Source: CAD feature listing. Evaluate the final solid. Frame: model axes, mm. A direction names the side the tool comes from. Give positions to 0.01 mm unless a question says otherwise; leave off trailing zeros. Order: outer loops, then holes, each group sorted by start corner. A loop starts at its lowest first (then second) coordinate and runs counter-clockwise, first axis right, second up. Notation, with made-up numbers: (-32, 43.5) -> (-15, 43.5) arc R13 ccw to (-15, 57.5) -> close; hole circle Ø5 at (12.25, 25.5). An arc over 180 degrees is marked (long way). Answer in a Markdown table with one row per item.
```python
from build123d import *

# Parameters (mm, degrees)
F0_W     = 127
F0_H     = 127
F1_DEPTH = 12.7
F2_R     = 4.826
F3_DEPTH = 25.4
F4_R     = 3.429
F4_R_2   = 3.4577066483
F5_DEPTH = 25.4


# Not quite as in the source:
# - a feature names something its author has since deleted; it is built from what else it names


with BuildPart() as f1:
    # F0 (on Top) → F1 (new body)
    with BuildSketch(Plane.XY):
        Rectangle(F0_W, F0_H)
    extrude(amount=F1_DEPTH)

    # F2 (on face) → F3 (cut)
    with BuildSketch(Plane.XY.offset(12.7)):
        with BuildLine():
            ThreePointArc((-10.8373346815, 7.9672162229), (-15.8950533343, 8.195276323), (-15.6669932342, 3.1375576702))
            ThreePointArc((-15.6669932342, 3.1375576702), (-12.0167906073, 2.664949958), (-10.0413841816, 5.7706071703))
            ThreePointArc((-10.0413841816, 5.7706071703), (-10.2465070332, 6.9387925717), (-10.8373346815, 7.9672162229))
        make_face()
        with BuildLine():
            ThreePointArc((3.429, 11.3502229887), (-0.1544617901, 14.7757423005), (-3.4150843134, 11.0416129887))
            ThreePointArc((-3.4150843134, 11.0416129887), (0, 7.9212229887), (3.4150843134, 11.0416129887))
            ThreePointArc((3.4150843134, 11.0416129887), (3.4255193118, 11.1957611986), (3.429, 11.3502229887))
        make_face()
        with BuildLine():
            ThreePointArc((16.8993841816, 5.7706071703), (14.638569583, 8.9944843187), (10.8373346815, 7.9672162229))
            ThreePointArc((10.8373346815, 7.9672162229), (11.0457150289, 3.3459380176), (15.6669932342, 3.1375576702))
            ThreePointArc((15.6669932342, 3.1375576702), (16.576041394, 4.317013596), (16.8993841816, 5.7706071703))
        make_face()
        with BuildLine():
            ThreePointArc((22.479, -7.6997770113), (21.3629869552, -5.1683480976), (18.74139, -4.2846926978))
            ThreePointArc((18.74139, -4.2846926978), (15.621, -7.6997770113), (18.74139, -11.1148613247))
            ThreePointArc((18.74139, -11.1148613247), (21.3629869552, -10.231205925), (22.479, -7.6997770113))
        make_face()
        with BuildLine():
            ThreePointArc((15.6669932342, -18.5371116928), (11.0457150289, -18.7454920402), (10.8373346815, -23.3667702455))
            ThreePointArc((10.8373346815, -23.3667702455), (14.638569583, -24.3940383413), (16.8993841816, -21.1701611929))
            ThreePointArc((16.8993841816, -21.1701611929), (16.576041394, -19.7165676186), (15.6669932342, -18.5371116928))
        make_face()
        with BuildLine():
            ThreePointArc((3.4150843134, -26.4411670113), (0, -23.3207770113), (-3.4150843134, -26.4411670113))
            ThreePointArc((-3.4150843134, -26.4411670113), (-0.1544617901, -30.1752963231), (3.429, -26.7497770113))
            ThreePointArc((3.429, -26.7497770113), (3.4255193118, -26.5953152212), (3.4150843134, -26.4411670113))
        make_face()
        with BuildLine():
            ThreePointArc((-10.0413841816, -21.1701611929), (-12.0167906073, -18.0645039805), (-15.6669932342, -18.5371116928))
            ThreePointArc((-15.6669932342, -18.5371116928), (-15.8950533343, -23.5948303456), (-10.8373346815, -23.3667702455))
            ThreePointArc((-10.8373346815, -23.3667702455), (-10.2465070332, -22.3383465943), (-10.0413841816, -21.1701611929))
        make_face()
        with BuildLine():
            ThreePointArc((-15.621, -7.6997770113), (-16.5185710863, -5.3867900561), (-18.74139, -4.2846926978))
            ThreePointArc((-18.74139, -4.2846926978), (-22.479, -7.6997770113), (-18.74139, -11.1148613247))
            ThreePointArc((-18.74139, -11.1148613247), (-16.5185710863, -10.0127639665), (-15.621, -7.6997770113))
        make_face()
        with Locations((0, -7.6997770113)):
            Circle(F2_R)
    extrude(amount=-F3_DEPTH, mode=Mode.SUBTRACT)

    # F4 (on face) → F5 (cut)
    with BuildSketch(Plane.XY.offset(12.7)):
        with Locations((0, 50.8)):
            Circle(F4_R)
        with Locations((27.94, -55.88)):
            Circle(F4_R)
        with Locations((50.8, -55.88)):
            Circle(F4_R)
        with Locations((-50.8, -55.88)):
            Circle(F4_R)
        with Locations((-27.94, -55.88)):
            Circle(F4_R)
        with Locations((-53.594, 50.8)):
            Circle(F4_R_2)
        with Locations((53.594, 50.8)):
            Circle(F4_R_2)
        with BuildLine():
            Line((-22.479, 54.229), (-35.814, 54.229))
            ThreePointArc((-35.814, 54.229), (-39.243, 50.8), (-35.814, 47.371))
            Line((-35.814, 47.371), (-22.479, 47.371))
            ThreePointArc((-22.479, 47.371), (-19.05, 50.8), (-22.479, 54.229))
        make_face()
        with BuildLine():
            ThreePointArc((35.814, 47.371), (39.243, 50.8), (35.814, 54.229))
            Line((35.814, 54.229), (22.479, 54.229))
            ThreePointArc((22.479, 54.229), (19.05, 50.8), (22.479, 47.371))
            Line((22.479, 47.371), (35.814, 47.371))
        make_face()
    extrude(amount=-F5_DEPTH, mode=Mode.SUBTRACT)


solid = f1.part
```
(1) Section query D-D (x = 20.5). Return the cut outline in (y, z), plus the area to 3 significant figures.
A:
| item | result |
|---|---|
| outline | (-63.5, 0) -> (-10.81, 0) -> (-10.81, 12.7) -> (-63.5, 12.7) -> close; (-4.59, 0) -> (48, 0) -> (48, 12.7) -> (-4.59, 12.7) -> close; (53.6, 0) -> (63.5, 0) -> (63.5, 12.7) -> (53.6, 12.7) -> close |
| area | 1,460 mm^2 |
(2) Access query for faces 5 (the flat face through (63.5, -1, 6)), 6 (the cylindrical face through (39.242, 50.725, 6.439)). Directions: +Z, -Z, +X, -X, +Y, -Y. A direction counts if a zero-diameter tool reaches every point of the face in a straight line with its end or side. Return the directions, or none.
A:
| item | result |
|---|---|
| face 5 | +Z, -Z, +X, +Y, -Y |
| face 6 | +Z, -Z |
(3) First-contact query: pin 1 Ø5.5 at (x, y) = (53.594, 50.8) entering from +Z. Flat tip, straight axial feed; report the tip coordinate or a pass-through.
A:
| item | result |
|---|---|
| pin 1 | passes through |
(4) Pull-direction query (Y, two-part tool) for faces 1 (the flat face through (-1, -63.5, 6)), 2 (the cylindrical face through (-28.39, -52.48, 6.44)), 3 (the flat face through (-63.5, -1, 6)), 4 (the flat face through (-1, 63.5, 6)); classes: +Y half, -Y half, draft (parallel to the pull), parting line (faces both ways), or undercut.
A:
| item | result |
|---|---|
| face 1 | -Y half |
| face 2 | undercut |
| face 3 | draft |
| face 4 | +Y half |
(5) Section query C-C (y = 50.8). Return the cut outline in (x, z), plus the area to 3 significant figures.
A:
| item | result |
|---|---|
| outline | (-63.5, 0) -> (-57.05, 0) -> (-57.05, 12.7) -> (-63.5, 12.7) -> close; (-50.14, 0) -> (-39.24, 0) -> (-39.24, 12.7) -> (-50.14, 12.7) -> close; (-19.05, 0) -> (-3.43, 0) -> (-3.43, 12.7) -> (-19.05, 12.7) -> close; (3.43, 0) -> (19.05, 0) -> (19.05, 12.7) -> (3.43, 12.7) -> close; (39.24, 0) -> (50.14, 0) -> (50.14, 12.7) -> (39.24, 12.7) -> close; (57.05, 0) -> (63.5, 0) -> (63.5, 12.7) -> (57.05, 12.7) -> close |
| area | 837 mm^2 |
(6) Section query A-A (x = 0). Return the cut outline in (y, z), plus the area to 3 significant figures.
A:
| item | result |
|---|---|
| outline | (-63.5, 0) -> (-30.18, 0) -> (-30.18, 12.7) -> (-63.5, 12.7) -> close; (-23.32, 0) -> (-12.53, 0) -> (-12.53, 12.7) -> (-23.32, 12.7) -> close; (-2.87, 0) -> (7.92, 0) -> (7.92, 12.7) -> (-2.87, 12.7) -> close; (14.78, 0) -> (47.37, 0) -> (47.37, 12.7) -> (14.78, 12.7) -> close; (54.23, 0) -> (63.5, 0) -> (63.5, 12.7) -> (54.23, 12.7) -> close |
| area | 1,230 mm^2 |
(7) Section query B-B (y = -55.88). Return the cut outline in (x, z), plus the area to 3 significant figures.
A:
| item | result |
|---|---|
| outline | (-63.5, 0) -> (-54.23, 0) -> (-54.23, 12.7) -> (-63.5, 12.7) -> close; (-47.37, 0) -> (-31.37, 0) -> (-31.37, 12.7) -> (-47.37, 12.7) -> close; (-24.51, 0) -> (24.51, 0) -> (24.51, 12.7) -> (-24.51, 12.7) -> close; (31.37, 0) -> (47.37, 0) -> (47.37, 12.7) -> (31.37, 12.7) -> close; (54.23, 0) -> (63.5, 0) -> (63.5, 12.7) -> (54.23, 12.7) -> close |
| area | 1,260 mm^2 |
(8) Ray query, probe 1 along Y at (x, z) = (27.94, 7.75); probe 2 along X at (y, z) = (4.5, 11.5); probe 3 along Y at (x, z) = (23.5, 2.75). Return the intervals inside material, ascending.
A:
| item | result |
|---|---|
| probe 1 | y = -63.5 to -59.31, -52.45 to 47.37, 54.23 to 63.5 |
| probe 2 | x = -63.5 to -16.66, -10.29 to 10.29, 16.66 to 63.5 |
| probe 3 | y = -63.5 to 47.37, 54.23 to 63.5 |
